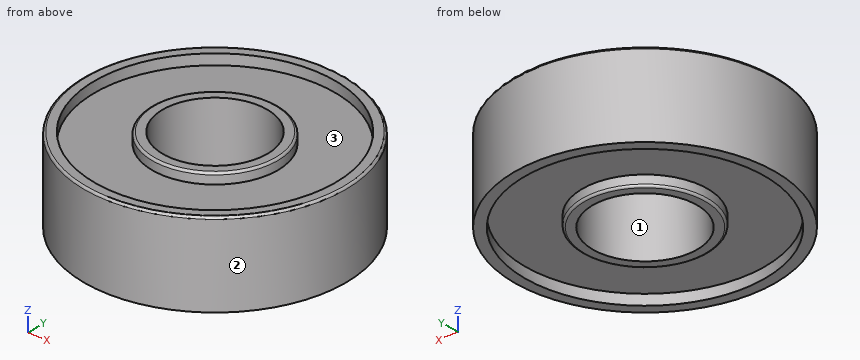
from build123d import *

# Parameters (mm, degrees)
F0_R     = 12.5
F1_DEPTH = 8
F2_R     = 5
F3_DEPTH = 8.001
F4_R     = 11.5
F4_R_2   = 6
F5_DEPTH = 1
F6_R     = 11.5
F6_R_2   = 6
F7_DEPTH = 1
F8_R     = 0.2


with BuildPart() as f1:
    # F0 (on Top) → F1 (new body)
    with BuildSketch(Plane.XY):
        Circle(F0_R)
    extrude(amount=F1_DEPTH)

    # F2 (on face) → F3 (cut, through all)
    with BuildSketch(Plane.XY.offset(8)):
        Circle(F2_R)
    extrude(amount=-F3_DEPTH, mode=Mode.SUBTRACT)

    # F4 (on face) → F5 (cut)
    with BuildSketch(Plane.XY.offset(8)):
        Circle(F4_R)
        Circle(F4_R_2, mode=Mode.SUBTRACT)
    extrude(amount=-F5_DEPTH, mode=Mode.SUBTRACT)

    # F6 (on face) → F7 (cut)
    with BuildSketch(Plane(origin=(0, 0, 0), x_dir=(1, 0, 0), z_dir=(0, 0, -1))):
        Circle(F6_R)
        Circle(F6_R_2, mode=Mode.SUBTRACT)
    extrude(amount=-F7_DEPTH, mode=Mode.SUBTRACT)

    # F8
    f8_edges = [f1.edges().sort_by_distance(p)[0] for p in [
        (-12.5, 0, 8),
        (-6, 0, 8),
        (-6, 0, 0),
    ]]
    fillet(f8_edges, radius=F8_R)


solid = f1.part
Source: CAD feature listing. Evaluate the final solid. Frame: model axes, mm. Face numbers are marked on the shaded views. Coordinates: 2 decimals unless noted, no trailing zeros. Loops run counter-clockwise (first coordinate to the right, second up) from the corner with the lowest first, then second, coordinate; pieces in that order, holes last. Notation, with made-up numbers: M 62.25,-6.75 L 84.25,-6.75 A26 ccw 84.25,17.25 Z; hole C 35.5,12 d10. An arc over 180 degrees is marked long. Answer in a Markdown table with one row per item.
Q1. First-contact query: pin 1 (1 mm diameter, centred on y = 7.5, z = 5.5, fed in from -X); pin 2 (1 mm diameter, centred on y = 9, z = 6, fed in from +X); pin 3 (4 mm diameter, centred on x = -9.5, z = 6, fed in from -Y). Flat tips, straight axial feed; report the tip coordinate or a pass-through.
Answers below:
| item | result |
|---|---|
| pin 1 | stops at x = -10.36 |
| pin 2 | stops at x = 9.17 |
| pin 3 | stops at y = -10 |
Q2. Section B-B on z = 0.5. Return the cut outline in (x, y).
Answers below:
| item | result |
|---|---|
| outline | C 0,0 d25; C 0,0 d12; hole C 0,0 d23; hole C 0,0 d10 |
Q3. Draft query along X for the marked faces 1, 2 and 3. Return one class per face: pulls with the +X half, pulls with the -X half, needs draft (parallel to the pull), parting line crosses it, or undercut.
Answers below:
| item | result |
|---|---|
| face 1 | undercut |
| face 2 | parting line crosses it |
| face 3 | undercut |
Q4. Ray query, probe 1 along Y at (x, z) = (0, 0.6); probe 2 along Y at (x, z) = (-1.5, 7.5); probe 3 along X at (y, z) = (0.25, 5). Return the intervals inside material, ascending. Write a range as from..to.
Answers below:
| item | result |
|---|---|
| probe 1 | y = -12.5..-11.5, -6..-5, 5..6, 11.5..12.5 |
| probe 2 | y = -12.41..-11.4, -5.81..-4.77, 4.77..5.81, 11.4..12.41 |
| probe 3 | x = -12.5..-4.99, 4.99..12.5 |
